Geometry check sheet. Reference: drawing and pictorial views, mm from the part's lowest x, y, z. Give positions to 0.01 mm unless a question says otherwise; leave off trailing zeros. Order: outer loops, then holes, each group sorted by start corner. A loop starts at its lowest first (then second) coordinate and runs counter-clockwise, first axis right, second up. Notation, with made-up numbers: M 41,71.5 L 51,71.5 A23 ccw 51,88.5 Z; hole C -27,-21 d3. An arc over 180 degrees is marked long. Answer as CSV lines item,"result".
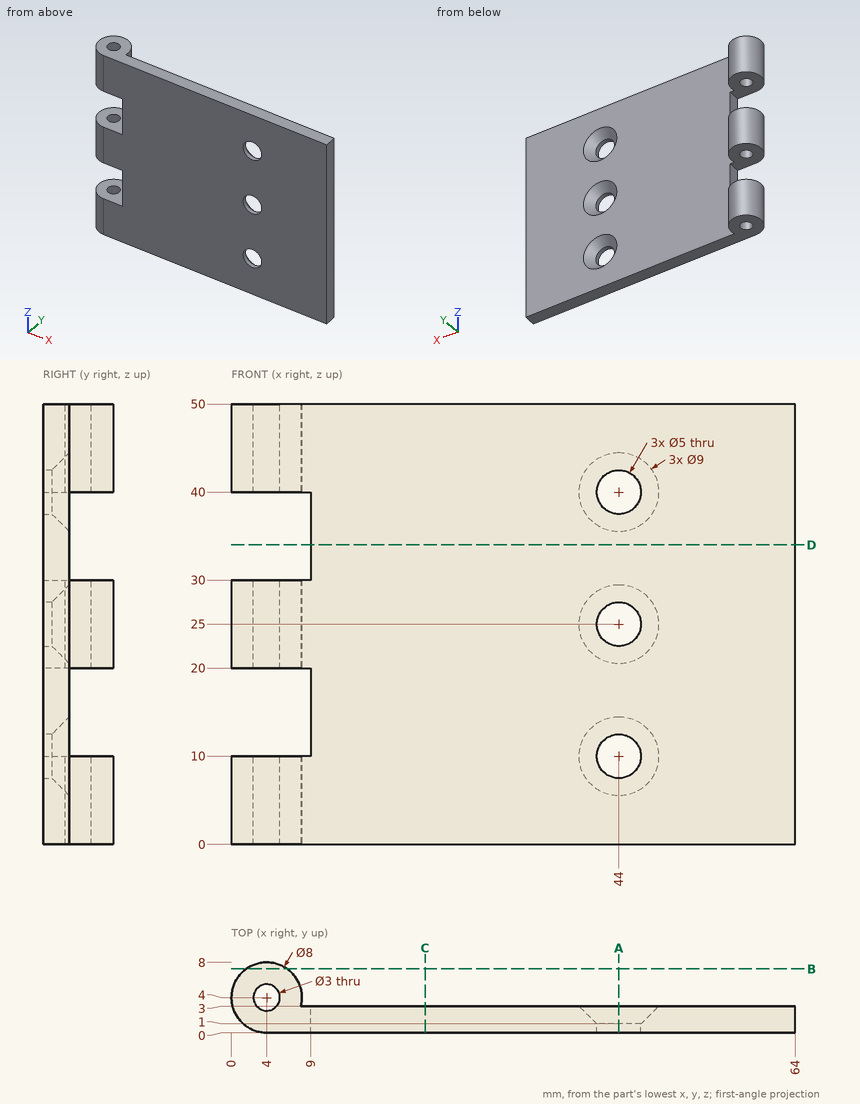
(1) Material ranges on line 1 (Y direction, x = 4, z = 2.75); line 2 (X direction, y = 1.5, z = 32.5); line 3 (Y direction, x = 26.5, z = 6.5), recorded low to high.
The answers:
line 1,"y = 0 to 2.5, 5.5 to 8"
line 2,"x = 9 to 64"
line 3,"y = 0 to 3"
(2) Section check C-C on x = 22. Enter the section's corners in (y, z), then the cut area to 3 significant figures.
The answers:
outline,"M 0,0 L 3,0 L 3,50 L 0,50 Z"
area,"150 mm2"
(3) Section check A-A on x = 44. Enter the section's corners in (y, z), then the cut area to 3 significant figures.
The answers:
outline,"M 0,0 L 3,0 L 3,5.5 L 1,7.5 L 0,7.5 Z; M 0,12.5 L 1,12.5 L 3,14.5 L 3,20.5 L 1,22.5 L 0,22.5 Z; M 0,27.5 L 1,27.5 L 3,29.5 L 3,35.5 L 1,37.5 L 0,37.5 Z; M 0,42.5 L 1,42.5 L 3,44.5 L 3,50 L 0,50 Z"
area,"93.0 mm2"
(4) Section check D-D on z = 34. Enter the section's corners in (x, y).
The answers:
outline,"M 9,0 L 64,0 L 64,3 L 9,3 Z"
(5) Section check B-B on y = 7.25. Enter the section's corners in (x, z).
The answers:
outline,"M 1.67,0 L 6.33,0 L 6.33,10 L 1.67,10 Z; M 1.67,20 L 6.33,20 L 6.33,30 L 1.67,30 Z; M 1.67,40 L 6.33,40 L 6.33,50 L 1.67,50 Z"
(6) Gauge pin test, flat ends, axial feed: P1, Ø6, axis at x = 44, z = 10, coming from the +Y side; P2, Ø12, axis at x = 17.5, z = 13.5, coming from the -Y side; P3, Ø1.5, axis at y = 1, z = 12.5, coming from the -X side; P4, Ø10, axis at x = 20.5, z = 15, coming from the +Y side. Record the tip position at first contact, or that the pin passes through.
The answers:
P1,"stops at y = 1.5"
P2,"stops at y = 0"
P3,"stops at x = 9"
P4,"stops at y = 3"
